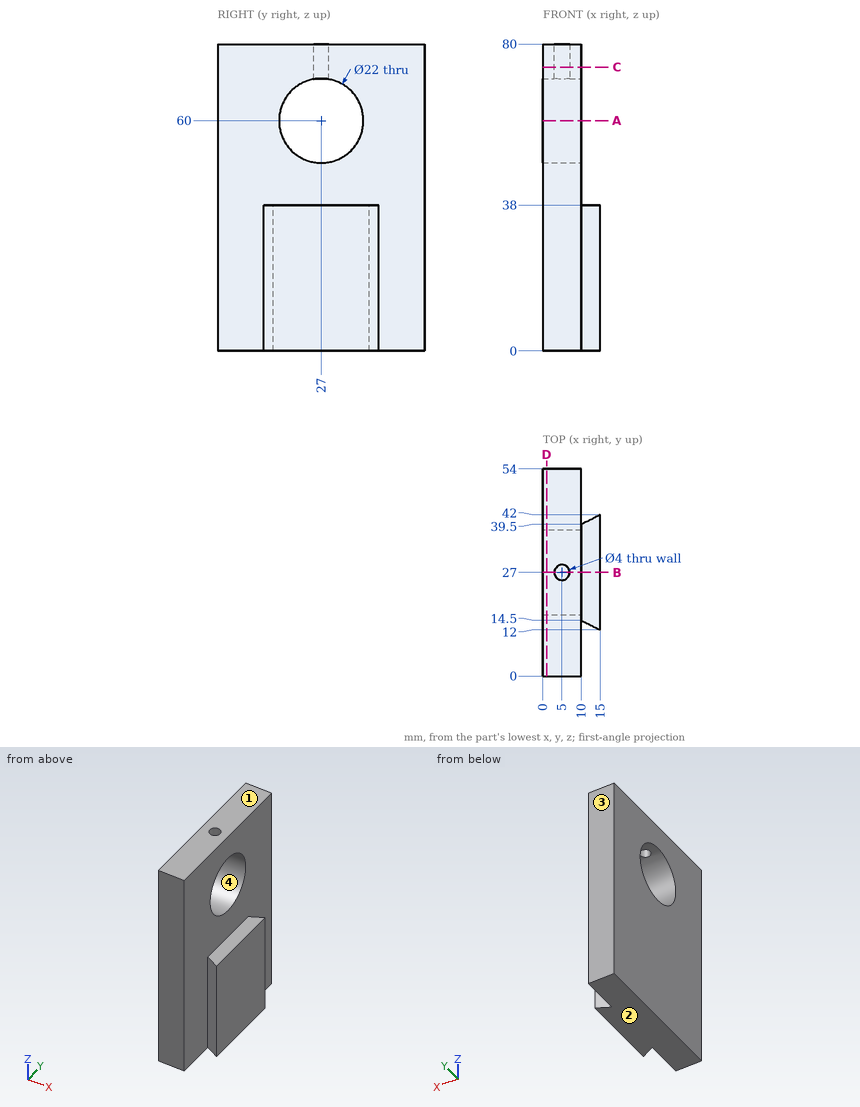
Input: dimensioned drawing with shaded views. Units: mm. Origin: part minimum x, y, z. Coordinates: 2 decimals unless noted, no trailing zeros. Order: outer loops, then holes, each group sorted by start corner. A loop starts at its lowest first (then second) coordinate and runs counter-clockwise, first axis right, second up. Notation, with made-up numbers: (-11, 62.5) -> (46, 62.5) arc R7 ccw to (46, 72.5) -> close; hole circle Ø9 at (-5, 19). An arc over 180 degrees is marked (long way). Answer in a Markdown table with one row per item.
Item 1: Section D-D on x = 1. Output: boundary loops of the cut face in (y, z), plus the area to 3 significant figures.
Return value:
| item | result |
|---|---|
| outline | (0, 0) -> (54, 0) -> (54, 80) -> (0, 80) -> close; hole circle Ø22 at (27, 60) |
| area | 3,940 mm² |
Item 2: Section B-B on y = 27. Output: boundary loops of the cut face in (x, z).
Return value:
| item | result |
|---|---|
| outline | (0, 0) -> (15, 0) -> (15, 38) -> (10, 38) -> (10, 49) -> (0, 49) -> close; (0, 71) -> (3, 71) -> (3, 80) -> (0, 80) -> close; (7, 71) -> (10, 71) -> (10, 80) -> (7, 80) -> close |
Item 3: Draft query along Z for the marked faces 1, 2, 3 and 4. Return one class per face: released by +Z, released by -Z, zero draft, split by the parting line, or undercut.
Return value:
| item | result |
|---|---|
| face 1 | released by +Z |
| face 2 | released by -Z |
| face 3 | zero draft |
| face 4 | undercut |
Item 4: Contact query for flat-ended pins moving along their axis: P1, Ø1.5, axis at x = 11.5, y = 32, coming from the +Z side; P2, Ø2, axis at y = 47.5, z = 65, coming from the +X side. Output: stop coordinate, or through.
Return value:
| item | result |
|---|---|
| P1 | stops at z = 38 |
| P2 | stops at x = 10 |
Item 5: Section C-C on z = 74. Output: boundary loops of the cut face in (x, y).
Return value:
| item | result |
|---|---|
| outline | (0, 0) -> (10, 0) -> (10, 54) -> (0, 54) -> close; hole circle Ø4 at (5, 27) |
Item 6: Ray query, L1, parallel to X at y = 27, z = 74; L2, parallel to Y at x = 5, z = 76.5; L3, parallel to Z at x = 2.5, y = 27. Return the intervals inside material, ascending.
Return value:
| item | result |
|---|---|
| L1 | x = 0 to 3, 7 to 10 |
| L2 | y = 0 to 25, 29 to 54 |
| L3 | z = 0 to 49, 71 to 80 |
Item 7: Section A-A on z = 60. Output: boundary loops of the cut face in (x, y).
Return value:
| item | result |
|---|---|
| outline | (0, 0) -> (10, 0) -> (10, 16) -> (0, 16) -> close; (0, 38) -> (10, 38) -> (10, 54) -> (0, 54) -> close |
